For this review, take the finished solid that the model builds, in its own axes (mm). A direction names the side the tool comes from. Coordinates: 2 decimals unless noted, no trailing zeros. Write each loop counter-clockwise with the first axis right and the second up, starting at its lowest first coordinate (ties: lowest second). Pieces come first, ordered by that corner, then holes. Notation, with made-up numbers: M -19,-18.75 L 24,-18.75 A14 cw 24,-0.75 Z; hole C 45,30 d7. An arc over 180 degrees is marked long. Return JSON: item names as keys, results as strings.
```python
from build123d import *

# Parameters (mm, degrees)
PAD_DEPTH       = 12
POCKET_DEPTH    = 3.65
SKETCH002_R     = 1.75
POCKET001_DEPTH = 5


with BuildPart() as part:
    # Sketch → Pad (new body)
    with BuildSketch(Plane.XY):
        with BuildLine():
            Line((-3.85, 8.2), (3.85, 8.2))
            Line((3.85, 8.2), (3.95, 7.75))
            Line((3.95, 7.75), (2.242615, 4.718526))
            ThreePointArc((0.5, 3.7), (1.50922, 3.973305), (2.242615, 4.718526))
            Line((0.5, 3.7), (-0.5, 3.7))
            ThreePointArc((-2.242615, 4.718526), (-1.50922, 3.973305), (-0.5, 3.7))
            Line((-2.242615, 4.718526), (-3.95, 7.75))
            Line((-3.85, 8.2), (-3.95, 7.75))
        make_face()
    extrude(amount=PAD_DEPTH)

    # Sketch001 (on Face7 of Pad) → Pocket (cut)
    with BuildSketch(Plane.XZ.offset(-3.7)):
        Polygon((-3.175426, 6), (-1.587713, 3.25), (1.587713, 3.25), (3.175426, 6), (1.587713, 8.75), (-1.587713, 8.75), align=None)
    extrude(amount=-POCKET_DEPTH, mode=Mode.SUBTRACT)

    # Sketch002 (on Face9 of Pocket) → Pocket001 (cut)
    with BuildSketch(Plane(origin=(0, 8.2, 0), x_dir=(-1, 0, 0), z_dir=(0, 1, 0))):
        with Locations((0, 6)):
            Circle(SKETCH002_R)
    extrude(amount=-POCKET001_DEPTH, mode=Mode.SUBTRACT)


solid = part.part
```
1. We need section B-B (y = 5.25). State the section outline as (x, z) points.
Checks:
{"outline": "M -2.54,0 L 2.54,0 L 2.54,4.9 L 1.59,3.25 L -1.59,3.25 L -2.54,4.9 Z; M -2.54,7.1 L -1.59,8.75 L 1.59,8.75 L 2.54,7.1 L 2.54,12 L -2.54,12 Z"}
2. Wall thickness on L1, parallel to Z at x = -1, y = 4.1; L2, parallel to Z at x = 0, y = 7.6; L3, parallel to Y at x = -1.25, z = 1: over which ranges is each line inside the solid? List them lowest first. Write a range as from..to.
Checks:
{"L1": "0..3.25, 8.75..12", "L2": "0..4.25, 7.75..12", "L3": "3.85..8.2"}
3. We need section A-A (z = 7.25). State the section outline as (x, y) points.
Checks:
{"outline": "M -3.95,7.75 L -2.45,5.09 L -2.45,7.35 L -1.22,7.35 L -1.22,8.2 L -3.85,8.2 Z; M 1.22,7.35 L 2.45,7.35 L 2.45,5.09 L 3.95,7.75 L 3.85,8.2 L 1.22,8.2 Z"}
4. We need section C-C (z = 10.75). State the section outline as (x, y) points.
Checks:
{"outline": "M -3.95,7.75 L -2.24,4.72 A2 ccw -0.5,3.7 L 0.5,3.7 A2 ccw 2.24,4.72 L 3.95,7.75 L 3.85,8.2 L -3.85,8.2 Z"}
5. Clearance check with flat-ended pins moving along their axes: pin 1 Ø1 at (y, z) = (5.5, 9) entering from +X; pin 2 Ø3 at (x, z) = (0, 6.5) entering from -Y; pin 3 Ø1 at (x, z) = (2, 1.5) entering from -Y. State where each tip first meets the part, or that it passes through.
Checks:
{"pin 1": "x = 2.96", "pin 2": "y = 7.35", "pin 3": "y = 3.97"}
6. We need section D-D (x = 2.5). State the section outline as (y, z) points, plus the area to 3 significant figures.
Checks:
{"outline": "M 5.18,0 L 8.2,0 L 8.2,12 L 5.18,12 L 5.18,7.17 L 7.35,7.17 L 7.35,4.83 L 5.18,4.83 Z", "area": "31.2 mm2"}
7. Draft analysis for pull direction Z (two halves, no side actions). For faces 3 (the face through (0, 6, 0)), 4 (the face through (1.5, 3.97, 1.67)), 5 (the face through (-2.216, 6.032, 4.339)), state which applies: +Z half, -Z half, draft (parallel to the pull), parting line (faces both ways), or undercut.
Checks:
{"face 3": "-Z half", "face 4": "draft", "face 5": "undercut"}
8. For faces 1 (the face through (1.5, 3.97, 10.26)), 2 (the face through (1.4, 7.35, 7.3)), list the 3-axis set-ups (+Z, -Z, +X, -X, +Y, -Y) from which the entire face can be reached by the end or side of a thin tool; tool diameter is ignored.
Checks:
{"face 1": "+Z, -Z, +X, -Y", "face 2": "-Y"}
